Geometry check sheet. Reference: the model listing, model coordinates, mm. Coordinates: 2 decimals unless noted, no trailing zeros.
from build123d import *

# Parameters (mm, degrees)
F0_W     = 1219.2
F0_H     = 609.6
F1_DEPTH = 6.35
F2_R     = 19.05
F3_DEPTH = 6.35
F4_R     = 12.7
F5_DEPTH = 6.35


with BuildPart() as f1:
    # F0 (on Top) → F1 (new body)
    with BuildSketch(Plane.XY):
        with Locations((609.6, 304.8)):
            Rectangle(F0_W, F0_H)
    extrude(amount=F1_DEPTH)

    # F2 (on face) → F3 (cut, through all)
    with BuildSketch(Plane.XY.offset(6.35)):
        with Locations((69.85, 539.75)):
            Circle(F2_R)
        with Locations((146.05, 539.75)):
            Circle(F2_R)
        with Locations((222.25, 539.75)):
            Circle(F2_R)
        with Locations((298.45, 539.75)):
            Circle(F2_R)
        with Locations((374.65, 539.75)):
            Circle(F2_R)
        with Locations((450.85, 539.75)):
            Circle(F2_R)
        with Locations((527.05, 539.75)):
            Circle(F2_R)
        with Locations((603.25, 539.75)):
            Circle(F2_R)
        with Locations((679.45, 539.75)):
            Circle(F2_R)
        with Locations((755.65, 539.75)):
            Circle(F2_R)
        with Locations((831.85, 539.75)):
            Circle(F2_R)
        with Locations((908.05, 539.75)):
            Circle(F2_R)
        with Locations((984.25, 539.75)):
            Circle(F2_R)
        with Locations((1060.45, 539.75)):
            Circle(F2_R)
        with Locations((1136.65, 539.75)):
            Circle(F2_R)
        with Locations((69.85, 463.55)):
            Circle(F2_R)
        with Locations((222.25, 463.55)):
            Circle(F2_R)
        with Locations((146.05, 463.55)):
            Circle(F2_R)
        with Locations((298.45, 463.55)):
            Circle(F2_R)
        with Locations((374.65, 463.55)):
            Circle(F2_R)
        with Locations((450.85, 463.55)):
            Circle(F2_R)
        with Locations((527.05, 463.55)):
            Circle(F2_R)
        with Locations((603.25, 463.55)):
            Circle(F2_R)
        with Locations((679.45, 463.55)):
            Circle(F2_R)
        with Locations((755.65, 463.55)):
            Circle(F2_R)
        with Locations((831.85, 463.55)):
            Circle(F2_R)
        with Locations((908.05, 463.55)):
            Circle(F2_R)
        with Locations((984.25, 463.55)):
            Circle(F2_R)
        with Locations((1060.45, 463.55)):
            Circle(F2_R)
        with Locations((1136.65, 463.55)):
            Circle(F2_R)
        with Locations((69.85, 387.35)):
            Circle(F2_R)
        with Locations((222.25, 387.35)):
            Circle(F2_R)
        with Locations((146.05, 387.35)):
            Circle(F2_R)
        with Locations((298.45, 387.35)):
            Circle(F2_R)
        with Locations((374.65, 387.35)):
            Circle(F2_R)
        with Locations((450.85, 387.35)):
            Circle(F2_R)
        with Locations((527.05, 387.35)):
            Circle(F2_R)
        with Locations((603.25, 387.35)):
            Circle(F2_R)
        with Locations((679.45, 387.35)):
            Circle(F2_R)
        with Locations((755.65, 387.35)):
            Circle(F2_R)
        with Locations((831.85, 387.35)):
            Circle(F2_R)
        with Locations((908.05, 387.35)):
            Circle(F2_R)
        with Locations((984.25, 387.35)):
            Circle(F2_R)
        with Locations((1060.45, 387.35)):
            Circle(F2_R)
        with Locations((1136.65, 387.35)):
            Circle(F2_R)
        with Locations((69.85, 311.15)):
            Circle(F2_R)
        with Locations((222.25, 311.15)):
            Circle(F2_R)
        with Locations((146.05, 311.15)):
            Circle(F2_R)
        with Locations((298.45, 311.15)):
            Circle(F2_R)
        with Locations((374.65, 311.15)):
            Circle(F2_R)
        with Locations((450.85, 311.15)):
            Circle(F2_R)
        with Locations((527.05, 311.15)):
            Circle(F2_R)
        with Locations((603.25, 311.15)):
            Circle(F2_R)
        with Locations((679.45, 311.15)):
            Circle(F2_R)
        with Locations((755.65, 311.15)):
            Circle(F2_R)
        with Locations((831.85, 311.15)):
            Circle(F2_R)
        with Locations((908.05, 311.15)):
            Circle(F2_R)
        with Locations((984.25, 311.15)):
            Circle(F2_R)
        with Locations((1060.45, 311.15)):
            Circle(F2_R)
        with Locations((1136.65, 311.15)):
            Circle(F2_R)
        with Locations((69.85, 234.95)):
            Circle(F2_R)
        with Locations((222.25, 234.95)):
            Circle(F2_R)
        with Locations((146.05, 234.95)):
            Circle(F2_R)
        with Locations((298.45, 234.95)):
            Circle(F2_R)
        with Locations((374.65, 234.95)):
            Circle(F2_R)
        with Locations((450.85, 234.95)):
            Circle(F2_R)
        with Locations((527.05, 234.95)):
            Circle(F2_R)
        with Locations((603.25, 234.95)):
            Circle(F2_R)
        with Locations((679.45, 234.95)):
            Circle(F2_R)
        with Locations((755.65, 234.95)):
            Circle(F2_R)
        with Locations((831.85, 234.95)):
            Circle(F2_R)
        with Locations((908.05, 234.95)):
            Circle(F2_R)
        with Locations((984.25, 234.95)):
            Circle(F2_R)
        with Locations((1060.45, 234.95)):
            Circle(F2_R)
        with Locations((1136.65, 234.95)):
            Circle(F2_R)
        with Locations((69.85, 158.75)):
            Circle(F2_R)
        with Locations((222.25, 158.75)):
            Circle(F2_R)
        with Locations((146.05, 158.75)):
            Circle(F2_R)
        with Locations((298.45, 158.75)):
            Circle(F2_R)
        with Locations((374.65, 158.75)):
            Circle(F2_R)
        with Locations((450.85, 158.75)):
            Circle(F2_R)
        with Locations((527.05, 158.75)):
            Circle(F2_R)
        with Locations((603.25, 158.75)):
            Circle(F2_R)
        with Locations((679.45, 158.75)):
            Circle(F2_R)
        with Locations((755.65, 158.75)):
            Circle(F2_R)
        with Locations((831.85, 158.75)):
            Circle(F2_R)
        with Locations((908.05, 158.75)):
            Circle(F2_R)
        with Locations((984.25, 158.75)):
            Circle(F2_R)
        with Locations((1060.45, 158.75)):
            Circle(F2_R)
        with Locations((1136.65, 158.75)):
            Circle(F2_R)
        with Locations((69.85, 82.55)):
            Circle(F2_R)
        with Locations((222.25, 82.55)):
            Circle(F2_R)
        with Locations((146.05, 82.55)):
            Circle(F2_R)
        with Locations((298.45, 82.55)):
            Circle(F2_R)
        with Locations((374.65, 82.55)):
            Circle(F2_R)
        with Locations((450.85, 82.55)):
            Circle(F2_R)
        with Locations((527.05, 82.55)):
            Circle(F2_R)
        with Locations((603.25, 82.55)):
            Circle(F2_R)
        with Locations((679.45, 82.55)):
            Circle(F2_R)
        with Locations((755.65, 82.55)):
            Circle(F2_R)
        with Locations((831.85, 82.55)):
            Circle(F2_R)
        with Locations((908.05, 82.55)):
            Circle(F2_R)
        with Locations((984.25, 82.55)):
            Circle(F2_R)
        with Locations((1060.45, 82.55)):
            Circle(F2_R)
        with Locations((1136.65, 82.55)):
            Circle(F2_R)
    extrude(amount=-F3_DEPTH, mode=Mode.SUBTRACT)

    # F4 (on face) → F5 (cut, through all)
    with BuildSketch(Plane.XY.offset(6.35)):
        with Locations((25.4, 584.2)):
            Circle(F4_R)
        with Locations((25.4, 25.4)):
            Circle(F4_R)
        with Locations((1193.8, 25.4)):
            Circle(F4_R)
        with Locations((1193.8, 584.2)):
            Circle(F4_R)
    extrude(amount=-F5_DEPTH, mode=Mode.SUBTRACT)


solid = f1.part
(1) Sectioned sample at A-A on x = 984.25. State how many separate pieces and enclosed holes the cut face has, and give its area (3 significant figures).
Findings:
separate pieces: 8
enclosed holes: 0
area: 2,180 mm2
(2) Gauge pin test, flat end, axial feed: pin 1 Ø23 at (x, y) = (755.65, 387.35) entering from -Z. Record the tip position at first contact, or that the pin passes through.
Findings:
pin 1: passes through
(3) Scan lines: L1, parallel to X at y = 584.2, z = 3.25; L2, parallel to X at y = 27, z = 3.75. Record each from-to range of solid material in increasing order.
Findings:
L1: x = 0 to 12.7, 38.1 to 1181.1, 1206.5 to 1219.2
L2: x = 0 to 12.8, 38 to 1181.2, 1206.4 to 1219.2
